Model file for the job. Use its own axes, mm. A direction names the side the tool comes from. Coordinates: 2 decimals unless noted, no trailing zeros. Write each loop counter-clockwise with the first axis right and the second up, starting at its lowest first coordinate (ties: lowest second). Pieces come first, ordered by that corner, then holes. Notation, with made-up numbers: M -2,-39 L 17,-39 A16 cw 17,-11 Z; hole C 56.5,-28.5 d3. An arc over 180 degrees is marked long. Use CSV: the item, a comma, the result in double quotes. Start each with the question number.
from build123d import *

# Parameters (mm, degrees)
SKETCH1_W               = 60
SKETCH1_H               = 35
SKETCH1_R               = 1.5
BOSS_EXTRUDE1_DEPTH     = 7
SKETCH5_R               = 7.5
BOSS_EXTRUDE5_DEPTH     = 3
SKETCH1_3_R             = 4
CUT_EXTRUDE1_DEPTH      = 3
CUT_EXTRUDE1_DEPTH_BACK = 3


with BuildPart() as part:
    # Sketch1 → Boss-Extrude1 (new body)
    with BuildSketch(Plane.XY):
        with Locations((-62.5, 0)):
            Rectangle(SKETCH1_W, SKETCH1_H)
        with Locations((-87.5, 12.5)):
            Circle(SKETCH1_R, mode=Mode.SUBTRACT)
        with Locations((-87.5, -12.5)):
            Circle(SKETCH1_R, mode=Mode.SUBTRACT)
        with Locations((-37.5, 12.5)):
            Circle(SKETCH1_R, mode=Mode.SUBTRACT)
        with Locations((-37.5, -12.5)):
            Circle(SKETCH1_R, mode=Mode.SUBTRACT)
    extrude(amount=BOSS_EXTRUDE1_DEPTH)

    # Sketch5 → Boss-Extrude5 (add)
    with BuildSketch(Plane.XY.offset(7)):
        with Locations((-62.5, 0)):
            Circle(SKETCH5_R)
    extrude(amount=BOSS_EXTRUDE5_DEPTH)

    # Sketch1_3 → Cut-Extrude1 (cut, two sides)
    with BuildSketch(Plane.XY) as cut_extrude1_sk:
        with Locations((-62.5, 0)):
            Circle(SKETCH1_3_R)
    extrude(amount=CUT_EXTRUDE1_DEPTH, mode=Mode.SUBTRACT)
    extrude(cut_extrude1_sk.sketch, amount=-CUT_EXTRUDE1_DEPTH_BACK, mode=Mode.SUBTRACT)


solid = part.part
1) Wall check: L1, parallel to Y at x = -37.5, z = 1.75; L2, parallel to Y at x = -88, z = 2.75; L3, parallel to Z at x = -89, y = 4. Give the ranges that are in metal, low to high. Write a range as [from, to].
2) Band-saw the part on A-A on y = -12.5. List the corners of the cut face in (x, z), then the cut area to 3 significant figures.
3) Two-plate mould, pull along X, no slides. Class faces 1 (the face through (-70, 0, 8)), 2 (the face through (-86.07, -12.05, 3.45)), 3 (the face through (-70, -4, 7)): pulls with the +X half, pulls with the -X half, needs draft (parallel to the pull), parting line crosses it, or undercut.
4) Band-saw the part on C-C on z = 2.25. List the corners of the cut face in (x, y), then the cut area to 3 significant figures.
5) Tool access for faces 4 (the face through (-63, 0, 3)), 5 (the face through (-62.92, 4.13, 0)): list every direction of +Z, -Z, +X, -X, +Y, -Y with a clear straight run to the whole face (end or side of a thin tool).
6) Band-saw the part on B-B on x = -37.5. List the corners of the cut face in (y, z), then the cut area to 3 significant figures.
7) Drop flat-ended pins along their axis: P1, Ø5, axis at x = -87.5, y = -12.5, coming from the +Z side; P2, Ø1, axis at x = -64, z = 8, coming from the -Y side. Give the stop position or say it passes through.
8) Band-saw the part on D-D on y = 0. List the corners of the cut face in (x, z), then the cut area to 3 significant figures.
Findings below:
1,L1,"y = [-17.5, -14], [-11, 11], [14, 17.5]"
1,L2,"y = [-17.5, -13.91], [-11.09, 11.09], [13.91, 17.5]"
1,L3,"z = [0, 7]"
2,outline,"M -92.5,0 L -89,0 L -89,7 L -92.5,7 Z; M -86,0 L -39,0 L -39,7 L -86,7 Z; M -36,0 L -32.5,0 L -32.5,7 L -36,7 Z"
2,area,"378 mm2"
3,face 1,"parting line crosses it"
3,face 2,"undercut"
3,face 3,"needs draft"
4,outline,"M -92.5,-17.5 L -32.5,-17.5 L -32.5,17.5 L -92.5,17.5 Z; hole C -87.5,-12.5 d3; hole C -87.5,12.5 d3; hole C -62.5,0 d8; hole C -37.5,-12.5 d3; hole C -37.5,12.5 d3"
4,area,"2,020 mm2"
5,face 4,"-Z"
5,face 5,"-Z, +X, -X, +Y, -Y"
6,outline,"M -17.5,0 L -14,0 L -14,7 L -17.5,7 Z; M -11,0 L 11,0 L 11,7 L -11,7 Z; M 14,0 L 17.5,0 L 17.5,7 L 14,7 Z"
6,area,"203 mm2"
7,P1,"stops at z = 7"
7,P2,"stops at y = -7.43"
8,outline,"M -92.5,0 L -66.5,0 L -66.5,3 L -58.5,3 L -58.5,0 L -32.5,0 L -32.5,7 L -55,7 L -55,10 L -70,10 L -70,7 L -92.5,7 Z"
8,area,"441 mm2"
